CAD build for the part. Positions are in the model's coordinates, mm. A direction names the side the tool comes from. Give positions to 0.01 mm unless a question says otherwise; leave off trailing zeros. Order: outer loops, then holes, each group sorted by start corner. A loop starts at its lowest first (then second) coordinate and runs counter-clockwise, first axis right, second up. Notation, with made-up numbers: M 41,43 L 70,43 A16 cw 70,67 Z; hole C 67,75.25 d5. An arc over 180 degrees is marked long. Put each result on its own line as item: value. Start each with the question number.
1) Pin check, flat tips, straight feed: pin 1 (0.9 mm diameter, centred on x = 46.5, y = 1, fed in from +Z); pin 2 (3 mm diameter, centred on x = 146, z = -4, fed in from -Y). Stop position of each tip, or through.
2) Cut at A-A (z = -86). Write the cut outline in (x, y).
3) Two-plate mould, pull along X, no slides. Class faces 4 (the face through (151, 1, -44)), 5 (the face through (0, 1, -44)), 6 (the face through (74, 1, -90)), 7 (the face through (64, 2, -53)): released by +X, released by -X, zero draft, split by the parting line, or undercut.
4) Tool access for faces 1 (the face through (22, 2, -72)), 2 (the face through (74, 3, -36)), 3 (the face through (107, 2, -22)): list every direction of +Z, -Z, +X, -X, +Y, -Y with a clear straight run to the whole face (end or side of a thin tool).
5) Cut at D-D (x = 6). Write the cut outline in (y, z).
6) Drill centre lines: line 1 (X direction, y = 2.4, z = -86); line 2 (X direction, y = 1.2, z = -4); line 3 (Z direction, x = 140, y = 1.8). Where is each one in solid material? Low to high. Write a range as [from, to].
7) Cut at C-C (z = -4). Write the cut outline in (x, y), and give its area (3 significant figures).
8) Cut at B-B (x = 70). Write the cut outline in (y, z), and give its area (3 significant figures).
```python
from build123d import *

# Parameters (mm, degrees)
SKETCH1_W           = 151
SKETCH1_H           = 90
BOSS_EXTRUDE1_DEPTH = 3
SKETCH2_R           = 1.75
CUT_EXTRUDE1_DEPTH  = 176.812400018
FILLET1_R           = 2
CUT_EXTRUDE2_DEPTH  = 176.812400018
FILLET2_R           = 2


with BuildPart() as part:
    # Sketch1 → Boss-Extrude1 (new body)
    with BuildSketch(Plane(origin=(0, 0, 0), x_dir=(1, 0, 0), z_dir=(0, 1, 0))):
        with Locations((75.5, 45)):
            Rectangle(SKETCH1_W, SKETCH1_H)
    extrude(amount=BOSS_EXTRUDE1_DEPTH)

    # Sketch2 → Cut-Extrude1 (cut, through all)
    with BuildSketch(Plane(origin=(0, 3, 0), x_dir=(1, 0, 0), z_dir=(0, 1, 0))):
        with Locations(Location((146, 86, 0), (0, 0, 270))):
            Circle(SKETCH2_R)
        with Locations(Location((146, 4, 0), (0, 0, 270))):
            Circle(SKETCH2_R)
        with Locations(Location((6, 86, 0), (0, 0, 270))):
            Circle(SKETCH2_R)
        with Locations(Location((6, 4, 0), (0, 0, 270))):
            Circle(SKETCH2_R)
    extrude(amount=-CUT_EXTRUDE1_DEPTH, mode=Mode.SUBTRACT)

    # Fillet1
    fillet1_edges = [part.edges().sort_by_distance(p)[0] for p in [
        (0, 1.5, -90),
        (151, 1.5, -90),
        (151, 1.5, 0),
        (0, 1.5, 0),
    ]]
    fillet(fillet1_edges, radius=FILLET1_R)

    # Sketch3 → Cut-Extrude2 (cut, through all)
    with BuildSketch(Plane(origin=(0, 3, 0), x_dir=(1, 0, 0), z_dir=(0, 1, 0))):
        Polygon((105, 62), (146, 62), (146, 82), (22, 82), (22, 62), (64, 62), (64, 43), (105, 43), align=None)
        Polygon((18, 0), (132, 0), (132, 15), (107, 15), (107, 29), (88, 29), (88, 15), (18, 15), align=None)
    extrude(amount=-CUT_EXTRUDE2_DEPTH, mode=Mode.SUBTRACT)

    # Fillet2
    fillet2_edges = [part.edges().sort_by_distance(p)[0] for p in [
        (18, 1.5, 0),
        (18, 1.5, -15),
        (88, 1.5, -15),
        (88, 1.5, -29),
        (107, 1.5, -29),
        (107, 1.5, -15),
        (132, 1.5, -15),
        (132, 1.5, 0),
    ]]
    fillet(fillet2_edges, radius=FILLET2_R)


solid = part.part
```
Solution:
1. pin 1: z = -15
1. pin 2: through
2. outline: M 0,0 L 4.25,0 L 4.25,3 L 0,3 Z; M 7.75,0 L 144.25,0 L 144.25,3 L 7.75,3 Z; M 147.75,0 L 151,0 L 151,3 L 147.75,3 Z
3. face 4: released by +X
3. face 5: released by -X
3. face 6: zero draft
3. face 7: undercut
4. face 1: +Y, -Y
4. face 2: +Z, -Z, +X, -X, +Y
4. face 3: +Z, +Y, -Y
5. outline: M 0,-90 L 3,-90 L 3,-87.75 L 0,-87.75 Z; M 0,-84.25 L 3,-84.25 L 3,-5.75 L 0,-5.75 Z; M 0,-2.25 L 3,-2.25 L 3,0 L 0,0 Z
6. line 1: [0, 4.25], [7.75, 144.25], [147.75, 151]
6. line 2: [0, 4.25], [7.75, 18], [132, 144.25], [147.75, 151]
6. line 3: [-90, -82], [-62, 0]
7. outline: M 0,0 L 4.25,0 L 4.25,3 L 0,3 Z; M 7.75,0 L 18,0 L 18,3 L 7.75,3 Z; M 132,0 L 144.25,0 L 144.25,3 L 132,3 Z; M 147.75,0 L 151,0 L 151,3 L 147.75,3 Z
7. area: 90.0 mm²
8. outline: M 0,-90 L 3,-90 L 3,-82 L 0,-82 Z; M 0,-43 L 3,-43 L 3,-15 L 0,-15 Z
8. area: 108 mm²
